from build123d import *

# Parameters (mm, degrees)
SKETCH1_W           = 76.498745459
SKETCH1_H           = 16.339745962
EXTRUDE1_DEPTH      = 2
SKETCH2_W           = 24.663668615
SKETCH2_H           = 16.339745962
EXTRUDE2_DEPTH      = 2
EXTRUDE3_DEPTH      = 16.339746
EXTRUDE4_DEPTH      = 2
EXTRUDE5_DEPTH      = 2
SKETCH6_W           = 24.021275531
SKETCH6_H           = 33.549299437
CUT_EXTRUDE2_DEPTH  = 5
SKETCH7_W           = 19.882310522
SKETCH7_H           = 22.758948474
CUT_EXTRUDE3_DEPTH  = 5
SKETCH8_W           = 89.248411888
SKETCH8_H           = 36.273905792
CUT_EXTRUDE4_DEPTH  = 5
SKETCH9_W           = 105.763953189
SKETCH9_H           = 17.720813838
CUT_EXTRUDE5_DEPTH  = 5
SKETCH10_W          = 34.758116025
SKETCH10_H          = 9.090411144
CUT_EXTRUDE6_DEPTH  = 5
SKETCH11_W          = 43.05920404
SKETCH11_H          = 32.49855368
CUT_EXTRUDE7_DEPTH  = 5
SKETCH12_W          = 30.563373624
SKETCH12_H          = 19.163652291
CUT_EXTRUDE8_DEPTH  = 5
CUT_EXTRUDE9_DEPTH  = 5
EXTRUDE6_REACH      = 127.538
SKETCH17_R          = 1.6
SKETCH18_R          = 3
CUT_EXTRUDE10_DEPTH = 46


with BuildPart() as part:
    # Sketch1 → Extrude1 (new body)
    with BuildSketch(Plane.XY):
        with Locations((24.172246601, 100.676372122)):
            Rectangle(SKETCH1_W, SKETCH1_H)
    extrude(amount=EXTRUDE1_DEPTH)



with BuildPart() as body_2:
    # Sketch2 → Extrude2 (new body)
    with BuildSketch(Plane(origin=(-0.816696373, 0, 3.834120606), x_dir=(0.9780578191404126, 0, 0.2083336324703724), z_dir=(-0.2083336324703724, -4.010680676458379e-15, 0.9780578191404126))):
        with Locations((-35.47509105, 100.676372122)):
            Rectangle(SKETCH2_W, SKETCH2_H)
    extrude(amount=EXTRUDE2_DEPTH)


with BuildPart() as part_1:
    add(part.part)

    add(body_2.part)  # Extrude3 merges body 2
    # Sketch3 → Extrude3 (add)
    with BuildSketch(Plane.XZ.offset(-92.506499141)):
        with BuildLine():
            Line((-14.077126129, 2), (-14.077126129, 0))
            ThreePointArc((-14.077126129, 0), (-18.790559922, -0.247530326), (-23.45213959, -0.987398139))
            Line((-23.45213959, -0.987398139), (-23.868806855, 0.9687175))
            ThreePointArc((-23.868806855, 0.9687175), (-19.000045868, 1.741468326), (-14.077126129, 2))
        make_face()
    extrude(amount=-EXTRUDE3_DEPTH)

    # Sketch4 → Extrude4 (add)
    with BuildSketch(Plane(origin=(0, 69.379874356, -40.056489136), x_dir=(1, 0, 0), z_dir=(1.6628191878975688e-14, -0.8660254037844406, 0.49999999999999695))):
        Polygon((48.995874099, 28.932741495), (66.339290827, 48.549555392), (-14.077126129, 48.549555392), (-14.077126129, 28.932741495), align=None)
    extrude(amount=EXTRUDE4_DEPTH)

    # Sketch5 → Extrude5 (add)
    with BuildSketch(Plane(origin=(8.140939792, 67.682405259, -38.219032255), x_dir=(0.9945598395247158, -0.09070455643384139, 0.0512192253622747), z_dir=(-0.1041668162351687, -0.866025403784443, 0.4890289095702023))):
        Polygon((-39.522656048, 25.582379856), (-28.623792922, 27.592891937), (-32.348610718, 47.784901585), (-60.160615909, 42.251632984), align=None)
    extrude(amount=EXTRUDE5_DEPTH)

    # Sketch6 → Cut-Extrude2 (cut)
    with BuildSketch(Plane(origin=(-24.396405636, 42.515816182, -2.71052281), x_dir=(0.867783590939769, 0.49593545163938957, -0.031617512598470475), z_dir=(0.4969422897034219, -0.8660254037844308, 0.05521196160555937))):
        with Locations((92.951842282, -1.018457271)):
            Rectangle(SKETCH6_W, SKETCH6_H)
    extrude(amount=CUT_EXTRUDE2_DEPTH, mode=Mode.SUBTRACT)

    # Sketch7 → Cut-Extrude3 (cut)
    with BuildSketch(Plane(origin=(61.660484884, 0, 6.850687483), x_dir=(0.11042392321111931, 2.1241172155137457e-15, -0.9938845794068167), z_dir=(0.9938845794068167, 1.91183874287404e-14, 0.11042392321111931))):
        with Locations((3.336054833, 99.931868434)):
            Rectangle(SKETCH7_W, SKETCH7_H)
    extrude(amount=CUT_EXTRUDE3_DEPTH, mode=Mode.SUBTRACT)

    # Sketch8 → Cut-Extrude4 (cut)
    with BuildSketch(Plane.XZ.offset(-83.846245103)):
        with Locations((7.257561645, -23.336285345)):
            Rectangle(SKETCH8_W, SKETCH8_H)
    extrude(amount=CUT_EXTRUDE4_DEPTH, mode=Mode.SUBTRACT)

    # Sketch9 → Cut-Extrude5 (cut)
    with BuildSketch(Plane.XY.offset(2)):
        with Locations((13.489075652, 93.672145699)):
            Rectangle(SKETCH9_W, SKETCH9_H)
    extrude(amount=CUT_EXTRUDE5_DEPTH, mode=Mode.SUBTRACT)

    # Sketch10 → Cut-Extrude6 (cut)
    with BuildSketch(Plane(origin=(-1.233363638, 0, 5.790236244), x_dir=(0.9780578191404125, 0, 0.2083336324703724), z_dir=(-0.20833363247037243, -4.0496183161323325e-15, 0.9780578191404126))):
        with Locations((-35.327877251, 93.473511189)):
            Rectangle(SKETCH10_W, SKETCH10_H)
    extrude(amount=CUT_EXTRUDE6_DEPTH, mode=Mode.SUBTRACT)

    # Sketch11 → Cut-Extrude7 (cut)
    with BuildSketch(Plane(origin=(-47.66681885, 0, -5.29594407), x_dir=(-0.11042392321111921, -2.1239244818946968e-15, 0.9938845794068167), z_dir=(-0.9938845794068167, -1.9116652705264417e-14, -0.11042392321111921))):
        with Locations((-0.835470819, 96.627603238)):
            Rectangle(SKETCH11_W, SKETCH11_H)
    extrude(amount=CUT_EXTRUDE7_DEPTH, mode=Mode.SUBTRACT)

    # Sketch12 → Cut-Extrude8 (cut)
    with BuildSketch(Plane(origin=(27.894822145, 48.612535322, 3.099208663), x_dir=(0.8677835909397874, -0.4959354516393574, -0.03161751259846775), z_dir=(-0.4969422897033898, -0.8660254037844495, -0.05521196160555938))):
        with Locations((-76.494352482, -16.060277262)):
            Rectangle(SKETCH12_W, SKETCH12_H)
    extrude(amount=CUT_EXTRUDE8_DEPTH, mode=Mode.SUBTRACT)

    # Sweep1: sweep along a curve in space
    with BuildLine() as sweep1_path:
        ThreePointArc((-23.45213959, 92.506499141, -0.987398139), (-18.790559922, 92.506499141, -0.247530326), (-14.077126129, 92.506499141, 0))
    # Sketch15 → Sweep1 (sweep)
    with BuildSketch(Plane(origin=(-22.635443217, 0, -4.821518744), x_dir=(0.2083336324703729, 4.064599859131597e-15, -0.9780578191404125), z_dir=(0.9780578191404125, 1.908195823574488e-14, 0.2083336324703729))):
        Polygon((-5.92013696, 92.506499141), (-5.92013696, 91.351798603), (7.07986304, 83.846245103), (11.07986304, 83.846245103), (-3.92013696, 92.506499141), align=None)
    sweep(path=sweep1_path.line)

    # Sketch16 → Cut-Extrude9 (cut)
    with BuildSketch(Plane(origin=(0, 67.647823548, -39.056489136), x_dir=(1, 0, 0), z_dir=(1.6740836018830237e-14, -0.8660254037844403, 0.4999999999999971))):
        with BuildLine():
            Line((-14.077126129, 24.677772288), (-14.077126129, 40.969683028))
            ThreePointArc((-14.077126129, 40.969683028), (-8.077126129, 46.969683028), (-2.077126129, 40.969683028))
            Line((-2.077126129, 40.969683028), (-2.077126129, 24.677772288))
            ThreePointArc((-2.077126129, 24.677772288), (-8.077126129, 18.677772288), (-14.077126129, 24.677772288))
        make_face()
    extrude(amount=-CUT_EXTRUDE9_DEPTH, mode=Mode.SUBTRACT)

    # Sketch17 → Extrude6 (add, up to next)
    with BuildSketch(Plane(origin=(1.202830139, 0, -10.826225801), x_dir=(0.9938845794068167, 0, 0.11042392321111931), z_dir=(-0.11042392321111931, -2.5465740627339532e-15, 0.9938845794068167)), mode=Mode.PRIVATE) as extrude6_sk1:
        with BuildLine():
            Line((-45.760115126, 98.553158182), (-45.760115126, 93.776669733))
            Line((-45.760115126, 93.776669733), (-40.803979116, 90.915243274))
            ThreePointArc((-40.803979116, 90.915243274), (-37.353292881, 98.581286318), (-45.760115126, 98.553158182))
        make_face()
        with Locations(Location((-41.547644752, 95.859630134, 0), (0, 0, 180))):
            Circle(SKETCH17_R, mode=Mode.SUBTRACT)
    extrude6_tool1 = extrude(extrude6_sk1.sketch, amount=EXTRUDE6_REACH, mode=Mode.PRIVATE) - part_1.part
    # Sketch17 → Extrude6 (add, up to next)
    with BuildSketch(Plane(origin=(1.202830139, 0, -10.826225801), x_dir=(0.9938845794068167, 0, 0.11042392321111931), z_dir=(-0.11042392321111931, -2.5465740627339532e-15, 0.9938845794068167)), mode=Mode.PRIVATE) as extrude6_sk2:
        with BuildLine():
            Line((59.839884874, 103.643328995), (59.839884874, 97.144098271))
            ThreePointArc((59.839884874, 97.144098271), (51.039884874, 100.393713633), (59.839884874, 103.643328995))
        make_face()
        with Locations((56.039884874, 100.393713633)):
            Circle(SKETCH17_R, mode=Mode.SUBTRACT)
    extrude6_tool2 = extrude(extrude6_sk2.sketch, amount=EXTRUDE6_REACH, mode=Mode.PRIVATE) - part_1.part
    add(extrude6_tool1.solids().sort_by_distance((-36.035052, 98.507498, -14.96348))[0])
    add(extrude6_tool2.solids().sort_by_distance((60.544377, 100.393714, -4.23318))[0])

    # Sketch18 → Cut-Extrude10 (cut)
    with BuildSketch(Plane(origin=(0.981982292, 0, -8.838456642), x_dir=(0.9938845794068167, 0, 0.11042392321111931), z_dir=(-0.11042392321111931, -2.5465740627339532e-15, 0.9938845794068167))):
        with Locations(Location((-41.547644752, 95.859630134, 0), (0, 0, 180))):
            Circle(SKETCH18_R)
        with Locations((56.039884874, 100.393713633)):
            Circle(SKETCH18_R)
    extrude(amount=CUT_EXTRUDE10_DEPTH, mode=Mode.SUBTRACT)


solid = part_1.part
CAD build for the part. Positions are in the model's coordinates, mm. A direction names the side the tool comes from. Coordinates: 2 decimals unless noted, no trailing zeros. Order: outer loops, then holes, each group sorted by start corner. A loop starts at its lowest first (then second) coordinate and runs counter-clockwise, first axis right, second up.
Item 1: 3-axis set-ups, long thin cutter, end or side, ignore diameter. For faces 1 (the face through (55.393, 99.353, -4.806)), 2 (the face through (-47.684, 100.791, -5.141)): which of +Z, -Z, +X, -X, +Y, -Y reach the whole face in a straight line?
Check sheet entries:
face 1: -Z, +X, +Y
face 2: -Z, -X, +Y, -Y
Item 2: Pin check, flat tips, straight feed: pin 1 Ø8 at (x, z) = (41, -11.5) entering from +Y; pin 2 Ø3 at (x, z) = (-23, 0) entering from -Y; pin 3 Ø1 at (y, z) = (99.5, -13.5) entering from +X. Stop position of each tip, or through.
Check sheet entries:
pin 1: stops at y = 88.18
pin 2: stops at y = 89.84
pin 3: stops at x = -36.38
Item 3: Two-plate mould, pull along Z, no slides. Class faces 3 (the face through (-2.077, 87, -8)), 4 (the face through (-18.72, 100.56, -0.24)), 5 (the face through (-18.369, 87.546, -4.82)), 6 (the face through (60.446, 100.439, -2.139)): +Z half, -Z half, draft (parallel to the pull), parting line (faces both ways), or undercut.
Check sheet entries:
face 3: draft
face 4: -Z half
face 5: +Z half
face 6: undercut
Item 4: Band-saw the part on A-A on x = 43. List the corners of the cut face in (y, z).
Check sheet entries:
outline: (83.85, -15) - (92.51, 0) - (108.85, 0) - (108.85, 2) - (91.35, 2) - (83.85, -11) - close
Item 5: Band-saw the part on B-B on z = -10. Give the number of separate pieces and of enclosed holes in the cut face, plus the area to 3 significant figures.
Check sheet entries:
separate pieces: 3
enclosed holes: 1
area: 226 mm2
Item 6: Drill centre lines: L1, parallel to Z at x = 34.5, y = 105; L2, parallel to Y at x = -13.5, z = -0.25; L3, parallel to Y at x = 17, z = 1.25. Where is each one in solid material? Low to high.
Check sheet entries:
L1: z = 0 to 2
L2: y = 90.05 to 92.36
L3: y = 90.92 to 108.85
